from build123d import *

# Parameters (mm, degrees)
SKETCH_1_R               = 40
EXTRUDE_1_DEPTH          = 15
EXTRUDE_2_DEPTH          = 15
PATTERN_CIRCULAR_1_COUNT = 20


with BuildPart() as part:
    # Sketch 1 → Extrude 1 (new body)
    with BuildSketch(Plane.XY):
        Circle(SKETCH_1_R)
    extrude(amount=EXTRUDE_1_DEPTH)

    # Sketch 2 → Extrude 2 (add)
    with BuildSketch(Plane.XY):
        Polygon((39.404775616, 3.709940518), (43.849373149, 4.41389561), (43.067200824, 9.352337313), (38.622603291, 8.648382221), align=None)
    extrude_2 = extrude(amount=EXTRUDE_2_DEPTH)

    # Pattern Circular 1: Extrude 2 ×20 about axis
    pattern_circular_1_axis = Axis((0, 0, 0), (0, 0, 1))
    for i in range(1, PATTERN_CIRCULAR_1_COUNT):
        add(extrude_2.rotate(pattern_circular_1_axis, i * 360 / PATTERN_CIRCULAR_1_COUNT))


solid = part.part
Verification items for the finished model (mm, model axes). A direction names the side the tool comes from. Coordinates: 2 decimals unless noted, no trailing zeros. Order: outer loops, then holes, each group sorted by start corner. A loop starts at its lowest first (then second) coordinate and runs counter-clockwise, first axis right, second up. Notation, with made-up numbers: M 73,0.5 L 114,0.5 A28 ccw 114,21.5 Z; hole C -33.5,5 d5. An arc over 180 degrees is marked long. Return JSON: item names as keys, results as strings.
1) Access from +Z, -Z, +X, -X, +Y, -Y to the whole of each face (thin tool, end or side, straight path). Record for faces 4 (the flat face through (4.1, 41.86, 7.4)), 5 (the flat face through (-16.835, -38.548, 7.395)), 6 (the flat face through (-38.5, -16.81, 7.4)).
Answer list:
{"face 4": "+Z, -Z, +Y", "face 5": "+Z, -Z, -Y", "face 6": "+Z, -Z, -X"}
2) Gauge pin test, flat ends, axial feed: pin 1 (8 mm diameter, centred on y = 3, z = 7.5, fed in from -X); pin 2 (1.5 mm diameter, centred on y = 10, z = 7.5, fed in from +X); pin 3 (8 mm diameter, centred on x = 17.5, z = 2, fed in from +Y). Record the tip position at first contact, or that the pin passes through.
Answer list:
{"pin 1": "x = -43.85", "pin 2": "x = 43.08", "pin 3": "y = 40.34"}
3) Thickness scan on L1, parallel to X at y = -31.5, z = 9.5; L2, parallel to X at y = 3.5, z = 1.75; L3, parallel to Y at x = 37, z = 10. Record the ranges inside material, lowest first. Write a range as [from, to].
Answer list:
{"L1": "[-30.73, -27.96], [-24.65, 24.65], [27.96, 30.73]", "L2": "[-39.85, 39.85]", "L3": "[-21.66, -16.05], [-15.2, 15.2], [16.05, 21.66]"}
4) Cross-section at A-A, the plane y = 24. Record the boundary of the cut face in (x, z), and give its area (3 significant figures).
Answer list:
{"outline": "M -32,0 L 32,0 L 32,15 L -32,15 Z", "area": "960 mm2"}
5) Cross-section at B-B, the plane x = 25. Record the boundary of the cut face in (y, z).
Answer list:
{"outline": "M -31.22,0 L 31.22,0 L 31.22,15 L -31.22,15 Z"}
6) Release check for a two-part mould opening along Y. For faces 1 (the flat face through (-1, 1, 0)), 2 (the flat face through (-19.944, 39.22, 7.395)), 3 (the flat face through (41.81, 4.09, 7.4)) record: +Y half, -Y half, draft (parallel to the pull), parting line (faces both ways), or undercut.
Answer list:
{"face 1": "draft", "face 2": "+Y half", "face 3": "undercut"}
